Here's the drawing with two shaded views (mm, measured from the low corner). I have some questions. Round coordinates to 2 decimals unless told otherwise and drop trailing zeros. Order: outer loops, then holes, each group sorted by start corner. A loop starts at its lowest first (then second) coordinate and runs counter-clockwise, first axis right, second up.
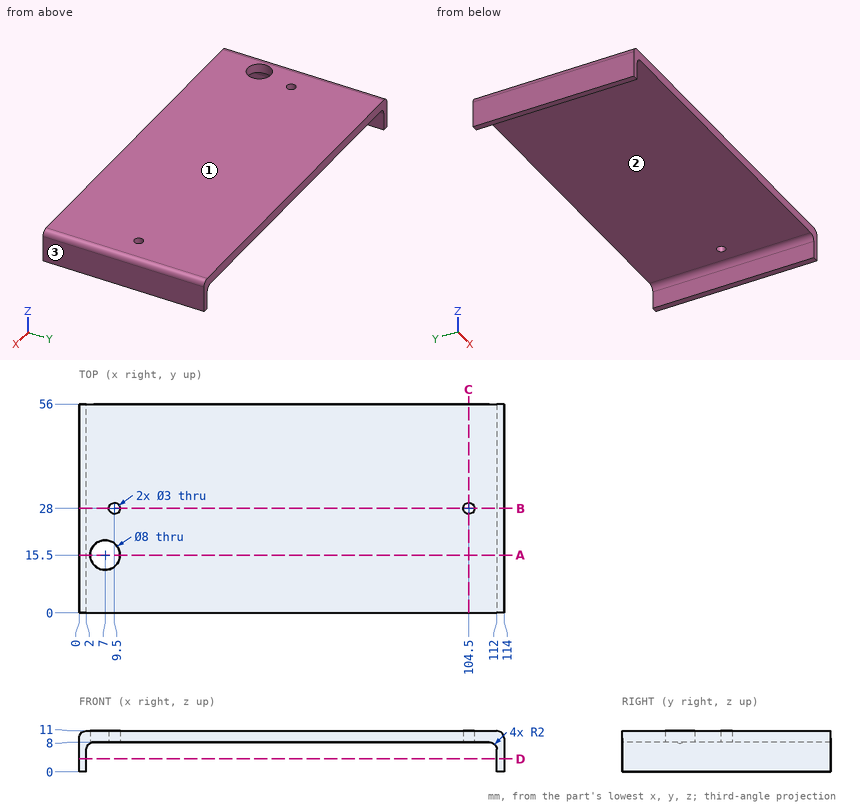
1. I need wall thicknesses on probe 1 along Y at (x, z) = (7, 8.4); probe 2 along Y at (x, z) = (104.5, 9.7); probe 3 along X at (y, z) = (51, 0.5). Which ranges of each line are inside material? Lowest first, please.
Evaluation:
probe 1: y = 0 to 11.5, 19.5 to 56
probe 2: y = 0 to 26.5, 29.5 to 56
probe 3: x = 0 to 2, 112 to 114
2. If we section it at B-B, the plane y = 28: Write out the boundary of the cut face in (x, z), and give its area (3 significant figures).
Evaluation:
outline: (0, 0) - (2, 0) - (2, 6) arc R2 cw to (4, 8) - (8, 8) - (8, 11) - (2, 11) arc R2 ccw to (0, 9) - close; (11, 8) - (103, 8) - (103, 11) - (11, 11) - close; (106, 8) - (110, 8) arc R2 cw to (112, 6) - (112, 0) - (114, 0) - (114, 9) arc R2 ccw to (112, 11) - (106, 11) - close
area: 356 mm2
3. If we mould it in two halves opening along Z, with no side actions, what happens to the marked faces 1, 2 and 3? For each: released by +Z, released by -Z, zero draft, split by the parting line, or undercut.
Evaluation:
face 1: released by +Z
face 2: released by -Z
face 3: zero draft
4. I'm going to push a flat-ended pin straight in: P1, Ø3, axis at x = 33, y = 32.5, coming from the -Z side. Where does the tip first touch, or does it pass through?
Evaluation:
P1: stops at z = 8
5. If we section it at A-A, the plane y = 15.5: Write out the boundary of the cut face in (x, z), and give its area (3 significant figures).
Evaluation:
outline: (0, 0) - (2, 0) - (2, 6) arc R2 cw to (3, 7.73) - (3, 11) - (2, 11) arc R2 ccw to (0, 9) - close; (11, 8) - (110, 8) arc R2 cw to (112, 6) - (112, 0) - (114, 0) - (114, 9) arc R2 ccw to (112, 11) - (11, 11) - close
area: 350 mm2
6. If we section it at D-D, the plane z = 3.5: Write out the boundary of the cut face in (x, y).
Evaluation:
outline: (0, 0) - (2, 0) - (2, 56) - (0, 56) - close; (112, 0) - (114, 0) - (114, 56) - (112, 56) - close
7. If we section it at C-C, the plane x = 104.5: Write out the boundary of the cut face in (y, z).
Evaluation:
outline: (0, 8) - (26.5, 8) - (26.5, 11) - (0, 11) - close; (29.5, 8) - (56, 8) - (56, 11) - (29.5, 11) - close
